Input: part model. Units: mm. Frame: model coordinates. A direction names the side the tool comes from. Give positions to 0.01 mm unless a question says otherwise; leave off trailing zeros. Order: outer loops, then holes, each group sorted by start corner. A loop starts at its lowest first (then second) coordinate and runs counter-clockwise, first axis right, second up. Notation, with made-up numbers: M 64.5,7.25 L 107.5,7.25 A10 ccw 107.5,17.25 Z; hole C 13.25,10 d10. An arc over 180 degrees is marked long. Use a Markdown table: item, result.
from build123d import *

# Parameters (mm, degrees)
SKETCH1_W           = 120
SKETCH1_H           = 67
BOSS_EXTRUDE1_DEPTH = 2
SKETCH2_R           = 5
BOSS_EXTRUDE2_DEPTH = 17
FILLET1_R           = 1
SKETCH3_W           = 25
SKETCH3_H           = 30
BOSS_EXTRUDE3_DEPTH = 47
SKETCH3_3_W         = 6
SKETCH3_3_H         = 40
BOSS_EXTRUDE4_DEPTH = 37
SKETCH3_4_W         = 5
SKETCH3_4_H         = 10
BOSS_EXTRUDE5_DEPTH = 17


with BuildPart() as part:
    # Sketch1 → Boss-Extrude1 (new body)
    with BuildSketch(Plane(origin=(0, 0, 0), x_dir=(1, 0, 0), z_dir=(0, 1, 0))):
        Rectangle(SKETCH1_W, SKETCH1_H)
    extrude(amount=BOSS_EXTRUDE1_DEPTH)

    # Sketch2 → Boss-Extrude2 (add)
    with BuildSketch(Plane(origin=(0, 2, 0), x_dir=(1, 0, 0), z_dir=(0, 1, 0))):
        with Locations((-53, 5.1)):
            Circle(SKETCH2_R)
        with Locations((-53, -5.1)):
            Circle(SKETCH2_R)
    extrude(amount=BOSS_EXTRUDE2_DEPTH)

    # Fillet1
    fillet1_edges = [part.edges().sort_by_distance(p)[0] for p in [
        (-58, 19, -5.1),
        (-58, 19, 5.1),
    ]]
    fillet(fillet1_edges, radius=FILLET1_R)

    # Sketch3 → Boss-Extrude3 (add)
    with BuildSketch(Plane(origin=(0, 2, 0), x_dir=(1, 0, 0), z_dir=(0, 1, 0))):
        with Locations((-17.5, 0)):
            Rectangle(SKETCH3_W, SKETCH3_H)
    extrude(amount=BOSS_EXTRUDE3_DEPTH)

    # Sketch3<3> → Boss-Extrude4 (add)
    with BuildSketch(Plane(origin=(0, 2, 0), x_dir=(1, 0, 0), z_dir=(0, 1, 0))):
        with Locations((15, 0)):
            Rectangle(SKETCH3_3_W, SKETCH3_3_H)
    extrude(amount=BOSS_EXTRUDE4_DEPTH)

    # Sketch3<4> → Boss-Extrude5 (add)
    with BuildSketch(Plane(origin=(0, 2, 0), x_dir=(1, 0, 0), z_dir=(0, 1, 0))):
        with Locations((37.5, 21.5)):
            Rectangle(SKETCH3_4_W, SKETCH3_4_H)
        with Locations((52.5, 21.5)):
            Rectangle(SKETCH3_4_W, SKETCH3_4_H)
    extrude(amount=BOSS_EXTRUDE5_DEPTH)


solid = part.part
1) Cut plane A-A on y = 32.5. Return loops of the section in (x, z), and give its area (3 significant figures).
Response values:
| item | result |
|---|---|
| outline | M -30,-15 L -5,-15 L -5,15 L -30,15 Z; M 12,-20 L 18,-20 L 18,20 L 12,20 Z |
| area | 990 mm² |
2) Cut plane B-B on y = 15. Return loops of the section in (x, z).
Response values:
| item | result |
|---|---|
| outline | C -53,-5.1 d10; C -53,5.1 d10; M -30,-15 L -5,-15 L -5,15 L -30,15 Z; M 12,-20 L 18,-20 L 18,20 L 12,20 Z; M 35,-26.5 L 40,-26.5 L 40,-16.5 L 35,-16.5 Z; M 50,-26.5 L 55,-26.5 L 55,-16.5 L 50,-16.5 Z |
3) Cut plane C-C on x = -24.5. Return loops of the section in (y, z), and give its area (3 significant figures).
Response values:
| item | result |
|---|---|
| outline | M 0,-33.5 L 2,-33.5 L 2,-15 L 49,-15 L 49,15 L 2,15 L 2,33.5 L 0,33.5 Z |
| area | 1,540 mm² |
4) Mould query, pull axis X, two halves, no side actions, for faces 1 (the face through (-30, 25, 0)), 2 (the face through (55, 10, -21)), 3 (the face through (-18, 49, 0)). Classes: released by +X, released by -X, zero draft, split by the parting line, or undercut.
Response values:
| item | result |
|---|---|
| face 1 | undercut |
| face 2 | released by +X |
| face 3 | zero draft |
5) Material intervals for line 1 (X direction, y = 27.5, z = -4.5); line 2 (X direction, y = 5.5, z = -20.5); line 3 (X direction, y = 32, z = -18), sorted ascending. Write a range as from..to.
Response values:
| item | result |
|---|---|
| line 1 | x = -30..-5, 12..18 |
| line 2 | x = 35..40, 50..55 |
| line 3 | x = 12..18 |
6) First-contact query: pin 1 Ø12 at (y, z) = (26, 11) entering from +X; pin 2 Ø3 at (x, y) = (14.5, 25) entering from +Z; pin 3 Ø1.5 at (x, y) = (37.5, 10.5) entering from -Z. Flat tips, straight axial feed; report the tip coordinate or a pass-through.
Response values:
| item | result |
|---|---|
| pin 1 | stops at x = 18 |
| pin 2 | stops at z = 20 |
| pin 3 | stops at z = -26.5 |
7) Reachability of faces 4 (the face through (15, 20, 20)), 5 (the face through (-58, 10, 5)), 6 (the face through (52, 10, -16.5)) from +Z, -Z, +X, -X, +Y, -Y: full face, straight path, thin tool, end or side. Return the list, or none.
Response values:
| item | result |
|---|---|
| face 4 | +Z, +X, -X, +Y |
| face 5 | +Y |
| face 6 | +Z, +X, +Y |
8) Cut plane D-D on z = -5.1. Return loops of the section in (x, y).
Response values:
| item | result |
|---|---|
| outline | M -60,0 L 60,0 L 60,2 L 18,2 L 18,39 L 12,39 L 12,2 L -5,2 L -5,49 L -30,49 L -30,2 L -48,2 L -48,18 A1 ccw -49,19 L -57,19 A1 ccw -58,18 L -58,2 L -60,2 Z |
